from build123d import *

# Parameters (mm, degrees)
SKETCH1_W           = 150
SKETCH1_H           = 150
SKETCH1_R           = 2.15
SKETCH1_R_2         = 2.65
BOSS_EXTRUDE1_DEPTH = 4
SKETCH2_R           = 2.65
BOSS_EXTRUDE2_DEPTH = 6
SKETCH3_R           = 4.5
SKETCH3_R_2         = 12.5
CUT_EXTRUDE1_DEPTH  = 6.5
SKETCH4_W           = 25
SKETCH4_H           = 25
CUT_EXTRUDE2_DEPTH  = 10
SKETCH5_W           = 37
SKETCH5_H           = 37
CUT_EXTRUDE3_DEPTH  = 6
SKETCH6_R           = 1.6
CUT_EXTRUDE4_DEPTH  = 24.5
CHAMFER1_SIZE       = 2
CUT_EXTRUDE5_DEPTH  = 24.5
CHAMFER2_SIZE       = 2
CHAMFER3_SIZE       = 0.5
CHAMFER4_SIZE       = 6


with BuildPart() as part:
    # Sketch1 → Boss-Extrude1 (new body)
    with BuildSketch(Plane(origin=(0, 0, 0), x_dir=(1, 0, 0), z_dir=(0, 1, 0))):
        with Locations((75, 75)):
            Rectangle(SKETCH1_W, SKETCH1_H)
        with Locations(Location((100, 142, 0), (0, 0, 270))):
            Circle(SKETCH1_R, mode=Mode.SUBTRACT)
        with Locations(Location((85, 142, 0), (0, 0, 270))):
            Circle(SKETCH1_R, mode=Mode.SUBTRACT)
        with Locations(Location((70, 142, 0), (0, 0, 270))):
            Circle(SKETCH1_R, mode=Mode.SUBTRACT)
        with Locations(Location((55, 142, 0), (0, 0, 270))):
            Circle(SKETCH1_R, mode=Mode.SUBTRACT)
        with Locations(Location((40, 142, 0), (0, 0, 270))):
            Circle(SKETCH1_R, mode=Mode.SUBTRACT)
        with Locations(Location((142, 40, 0), (0, 0, 270))):
            Circle(SKETCH1_R, mode=Mode.SUBTRACT)
        with Locations(Location((142, 55, 0), (0, 0, 270))):
            Circle(SKETCH1_R, mode=Mode.SUBTRACT)
        with Locations(Location((142, 70, 0), (0, 0, 270))):
            Circle(SKETCH1_R, mode=Mode.SUBTRACT)
        with Locations(Location((142, 85, 0), (0, 0, 270))):
            Circle(SKETCH1_R, mode=Mode.SUBTRACT)
        with Locations(Location((142, 100, 0), (0, 0, 270))):
            Circle(SKETCH1_R, mode=Mode.SUBTRACT)
        with Locations(Location((10, 30, 0), (0, 0, 270))):
            Circle(SKETCH1_R_2, mode=Mode.SUBTRACT)
        with Locations(Location((10, 80, 0), (0, 0, 270))):
            Circle(SKETCH1_R_2, mode=Mode.SUBTRACT)
        with Locations(Location((10, 130, 0), (0, 0, 270))):
            Circle(SKETCH1_R_2, mode=Mode.SUBTRACT)
        with Locations(Location((30, 10, 0), (0, 0, 270))):
            Circle(SKETCH1_R_2, mode=Mode.SUBTRACT)
        with Locations(Location((80, 10, 0), (0, 0, 270))):
            Circle(SKETCH1_R_2, mode=Mode.SUBTRACT)
        with Locations(Location((130, 10, 0), (0, 0, 270))):
            Circle(SKETCH1_R_2, mode=Mode.SUBTRACT)
    extrude(amount=BOSS_EXTRUDE1_DEPTH)

    # Sketch2 → Boss-Extrude2 (add)
    with BuildSketch(Plane(origin=(0, 4, 0), x_dir=(1, 0, 0), z_dir=(0, 1, 0))):
        Polygon((0, 150), (20, 150), (150, 150), (150, 134), (150, 20), (150, 0), (0, 0), align=None)
        with Locations(Location((10, 130, 0), (0, 0, 270))):
            Circle(SKETCH2_R, mode=Mode.SUBTRACT)
        with Locations(Location((10, 80, 0), (0, 0, 270))):
            Circle(SKETCH2_R, mode=Mode.SUBTRACT)
        with Locations(Location((10, 30, 0), (0, 0, 270))):
            Circle(SKETCH2_R, mode=Mode.SUBTRACT)
        with Locations(Location((30, 10, 0), (0, 0, 270))):
            Circle(SKETCH2_R, mode=Mode.SUBTRACT)
        with Locations(Location((80, 10, 0), (0, 0, 270))):
            Circle(SKETCH2_R, mode=Mode.SUBTRACT)
        with Locations(Location((130, 10, 0), (0, 0, 270))):
            Circle(SKETCH2_R, mode=Mode.SUBTRACT)
        Polygon((20, 134), (20, 20), (134, 20), (134, 109), (109, 109), (109, 134), align=None, mode=Mode.SUBTRACT)
        Polygon((59.099186911, 142), (57.049593456, 145.55), (52.950406544, 145.55), (50.900813089, 142), (52.950406544, 138.45), (57.049593456, 138.45), align=None, mode=Mode.SUBTRACT)
        Polygon((44.099186911, 142), (42.049593456, 145.55), (37.950406544, 145.55), (35.900813089, 142), (37.950406544, 138.45), (42.049593456, 138.45), align=None, mode=Mode.SUBTRACT)
        Polygon((74.099186911, 142), (72.049593456, 145.55), (67.950406544, 145.55), (65.900813089, 142), (67.950406544, 138.45), (72.049593456, 138.45), align=None, mode=Mode.SUBTRACT)
        Polygon((89.099186911, 142), (87.049593456, 145.55), (82.950406544, 145.55), (80.900813089, 142), (82.950406544, 138.45), (87.049593456, 138.45), align=None, mode=Mode.SUBTRACT)
        Polygon((104.099186911, 142), (102.049593456, 145.55), (97.950406544, 145.55), (95.900813089, 142), (97.950406544, 138.45), (102.049593456, 138.45), align=None, mode=Mode.SUBTRACT)
        Polygon((142, 80.900813089), (145.55, 82.950406544), (145.55, 87.049593456), (142, 89.099186911), (138.45, 87.049593456), (138.45, 82.950406544), align=None, mode=Mode.SUBTRACT)
        Polygon((142, 95.900813089), (145.55, 97.950406544), (145.55, 102.049593456), (142, 104.099186911), (138.45, 102.049593456), (138.45, 97.950406544), align=None, mode=Mode.SUBTRACT)
        Polygon((142, 65.900813089), (145.55, 67.950406544), (145.55, 72.049593456), (142, 74.099186911), (138.45, 72.049593456), (138.45, 67.950406544), align=None, mode=Mode.SUBTRACT)
        Polygon((142, 50.900813089), (145.55, 52.950406544), (145.55, 57.049593456), (142, 59.099186911), (138.45, 57.049593456), (138.45, 52.950406544), align=None, mode=Mode.SUBTRACT)
        Polygon((142, 35.900813089), (145.55, 37.950406544), (145.55, 42.049593456), (142, 44.099186911), (138.45, 42.049593456), (138.45, 37.950406544), align=None, mode=Mode.SUBTRACT)
    extrude(amount=BOSS_EXTRUDE2_DEPTH)

    # Sketch3 → Cut-Extrude1 (cut)
    with BuildSketch(Plane.XZ):
        with Locations(Location((10, -130, 0), (0, 0, 270))):
            Circle(SKETCH3_R)
        with Locations(Location((10, -80, 0), (0, 0, 270))):
            Circle(SKETCH3_R)
        with Locations(Location((10, -30, 0), (0, 0, 270))):
            Circle(SKETCH3_R)
        with Locations(Location((30, -10, 0), (0, 0, 270))):
            Circle(SKETCH3_R)
        with Locations(Location((80, -10, 0), (0, 0, 270))):
            Circle(SKETCH3_R)
        with Locations(Location((130, -10, 0), (0, 0, 270))):
            Circle(SKETCH3_R)
        with Locations(Location((65.625, -65.625, 0), (0, 0, 270))):
            Circle(SKETCH3_R_2)
    extrude(amount=-CUT_EXTRUDE1_DEPTH, mode=Mode.SUBTRACT)

    # Sketch4 → Cut-Extrude2 (cut)
    with BuildSketch(Plane(origin=(0, 10, 0), x_dir=(1, 0, 0), z_dir=(0, 1, 0))):
        with Locations((137.5, 137.5)):
            Rectangle(SKETCH4_W, SKETCH4_H)
    extrude(amount=-CUT_EXTRUDE2_DEPTH, mode=Mode.SUBTRACT)

    # Sketch5 → Cut-Extrude3 (cut)
    with BuildSketch(Plane(origin=(0, 10, 0), x_dir=(1, 0, 0), z_dir=(0, 1, 0))):
        with Locations((131.5, 131.5)):
            Rectangle(SKETCH5_W, SKETCH5_H)
    extrude(amount=-CUT_EXTRUDE3_DEPTH, mode=Mode.SUBTRACT)

    # Sketch6 → Cut-Extrude4 (cut)
    with BuildSketch(Plane(origin=(0, 4, 0), x_dir=(1, 0, 0), z_dir=(0, 1, 0))):
        with Locations(Location((119, 134.5, 0), (0, 0, 270))):
            Circle(SKETCH6_R)
        with Locations(Location((134.5, 119, 0), (0, 0, 270))):
            Circle(SKETCH6_R)
    extrude(amount=-CUT_EXTRUDE4_DEPTH, mode=Mode.SUBTRACT)

    # Chamfer1
    chamfer1_edges = [part.edges().sort_by_distance(p)[0] for p in [
        (75, 0, 0),
        (0, 0, -75),
    ]]
    chamfer(chamfer1_edges, length=CHAMFER1_SIZE)

    # Sketch7 → Cut-Extrude5 (cut)
    with BuildSketch(Plane.XZ):
        with BuildLine():
            Line((104, -71), (104, -56))
            ThreePointArc((104, -56), (110, -50), (116, -56))
            Line((116, -56), (116, -71))
            ThreePointArc((116, -71), (110, -77), (104, -71))
        make_face()
    extrude(amount=-CUT_EXTRUDE5_DEPTH, mode=Mode.SUBTRACT)

    # Chamfer2
    chamfer2_edges = [part.edges().sort_by_distance(p)[0] for p in [
        (65.625, 0, -53.125),
        (110, 0, -77),
        (116, 0, -63.5),
        (110, 0, -50),
        (104, 0, -63.5),
    ]]
    chamfer(chamfer2_edges, length=CHAMFER2_SIZE)

    # Chamfer3
    chamfer3_edges = [part.edges().sort_by_distance(p)[0] for p in [
        (125, 2, -150),
        (150, 2, -125),
    ]]
    chamfer(chamfer3_edges, length=CHAMFER3_SIZE)

    # Chamfer4
    chamfer4_edges = [part.edges().sort_by_distance(p)[0] for p in [
        (125, 2, -125),
    ]]
    chamfer(chamfer4_edges, length=CHAMFER4_SIZE)


solid = part.part
Model file for the job. Use its own axes, mm. A direction names the side the tool comes from. Coordinates: 2 decimals unless noted, no trailing zeros. Order: outer loops, then holes, each group sorted by start corner. A loop starts at its lowest first (then second) coordinate and runs counter-clockwise, first axis right, second up. Notation, with made-up numbers: M 3,-38 L 18,-38 A18 ccw 18,-33 Z; hole C 47.5,-33.75 d3. An arc over 180 degrees is marked long. Return JSON: item names as keys, results as strings.
1. Flat gauge pins, fed straight in: pin 1 (5 mm diameter, centred on x = 131, y = 7.5, fed in from -Z); pin 2 (7 mm diameter, centred on x = 55, z = -142, fed in from +Y); pin 3 (2.5 mm diameter, centred on x = 12, z = -31.5, fed in from -Y). Where does each tip first touch, or does it go through?
Ans:
{"pin 1": "z = -113", "pin 2": "y = 4", "pin 3": "y = 6.5"}
2. Drill centre lines: probe 1 along X at (y, z) = (2.75, -10); probe 2 along Z at (x, y) = (10, 8.8); probe 3 along X at (y, z) = (8, -10). Where is each one in solid material? Low to high.
Ans:
{"probe 1": "0 to 25.5, 34.5 to 75.5, 84.5 to 125.5, 134.5 to 150", "probe 2": "-150 to -132.65, -127.35 to -82.65, -77.35 to -32.65, -27.35 to 0", "probe 3": "0 to 27.35, 32.65 to 77.35, 82.65 to 127.35, 132.65 to 150"}
3. Pull direction Z, two halves, no side cores. Call faces 1 (the face through (145.55, 7, -55)), 2 (the face through (140, 4, -68)), 3 (the face through (76, 6, 0)): +Z half, -Z half, draft (parallel to the pull), parting line (faces both ways), or undercut.
Ans:
{"face 1": "undercut", "face 2": "undercut", "face 3": "+Z half"}
4. Saw through at B-B (x = 10). Give the number of separate pieces and of enclosed holes in the cut face, and give its area (3 significant figures).
Ans:
{"separate pieces": "4", "enclosed holes": "0", "area": "1,270 mm^2"}
5. Tool access for faces 4 (the face through (26.01, 3.2, -12.08)), 5 (the face through (78.02, 2.99, -64)), 6 (the face through (145.55, 7, -40)): list every direction of +Z, -Z, +X, -X, +Y, -Y with a clear straight run to the whole face (end or side of a thin tool).
Ans:
{"face 4": "-Y", "face 5": "+Y, -Y", "face 6": "+Y"}
6. Saw through at D-D (z = -30). Give the cut face in (x, y).
Ans:
{"outline": "M 0,2 L 2,0 L 5.5,0 L 5.5,6.5 L 7.35,6.5 L 7.35,10 L 0,10 Z; M 12.65,6.5 L 14.5,6.5 L 14.5,0 L 150,0 L 150,10 L 134,10 L 134,4 L 20,4 L 20,10 L 12.65,10 Z"}
7. Saw through at A-A (z = -100). Give the cut face in (x, y).
Ans:
{"outline": "M 0,2 L 2,0 L 139.85,0 L 139.85,4 L 138.45,4 L 138.45,10 L 134,10 L 134,4 L 20,4 L 20,10 L 0,10 Z; M 144.15,0 L 150,0 L 150,10 L 145.55,10 L 145.55,4 L 144.15,4 Z"}
